Here's how the part is built. I have some questions about the finished solid (model axes, mm). A direction names the side the tool comes from. Coordinates: 2 decimals unless noted, no trailing zeros. Write each loop counter-clockwise with the first axis right and the second up, starting at its lowest first coordinate (ties: lowest second). Pieces come first, ordered by that corner, then holes. Notation, with made-up numbers: (43.25, 26.5) -> (61.25, 26.5) arc R24 cw to (61.25, 43.5) -> close; hole circle Ø4 at (-32.5, 74.25). An arc over 180 degrees is marked (long way). Answer in a Markdown table with one row per item. Add a question column.
from build123d import *

# Parameters (mm, degrees)
BOSS_EXTRUDE1_DEPTH          = 30
EDGE_FLANGE1_STRIP_CUT_DEPTH = 30
EDGE_FLANGE1_DEPTH           = 30
EDGE_FLANGE2_STRIP_CUT_DEPTH = 30
EDGE_FLANGE2_DEPTH           = 30


# Sheet-metal steps are written as plain solids
with BuildPart() as part:
    # Sketch1 → Boss-Extrude1 (new body)
    with BuildSketch(Plane(origin=(0, 0, 0), x_dir=(0, 0, -1), z_dir=(1, 0, 0))):
        Polygon((0.196961551, -0.034729636), (8.879370434, 49.205658015), (8.485447333, 49.275117286), (-0.196961551, 0.034729636), align=None)
    extrude(amount=BOSS_EXTRUDE1_DEPTH)

    # Edge-Flange1 strip (across the edge) → Edge-Flange1 strip cut (cut)
    with BuildSketch(Plane(origin=(30, 49.275117286, -8.485447333), x_dir=(0, 0, 1), z_dir=(-1, 0, 0))):
        Polygon((-0.804601829, 2.259615531), (-0.387846202, -0.103923077), (0.006076899, -0.034463806), (-0.410678728, 2.329074802), align=None)
    extrude(amount=EDGE_FLANGE1_STRIP_CUT_DEPTH, mode=Mode.SUBTRACT)

    # Edge-Flange1 section (across the edge) → Edge-Flange1 (add)
    with BuildSketch(Plane(origin=(30, 49.275117286, -8.485447333), x_dir=(0, 0, 1), z_dir=(-1, 0, 0))):
        with BuildLine():
            Line((-0.4, 0.034995465), (-0.4, 2.965004535))
            Line((-0.4, 2.965004535), (0, 2.965004535))
            Line((0, 2.965004535), (0, 0.034995465))
            ThreePointArc((0, 0.034995465), (0.001522121, 0.000133168), (0.006076899, -0.034463806))
            Line((0.006076899, -0.034463806), (-0.387846202, -0.103923077))
            ThreePointArc((-0.387846202, -0.103923077), (-0.396955758, -0.034729129), (-0.4, 0.034995465))
        make_face()
    extrude(amount=EDGE_FLANGE1_DEPTH)

    # Edge-Flange2 strip (across the edge) → Edge-Flange2 strip cut (cut)
    with BuildSketch(Plane(origin=(30, -0.034729636, -0.196961551), x_dir=(0, 0, -1), z_dir=(-1, 0, 0))):
        Polygon((-0.804601829, 2.259615531), (-0.387846202, -0.103923077), (0.006076899, -0.034463806), (-0.410678728, 2.329074802), align=None)
    extrude(amount=EDGE_FLANGE2_STRIP_CUT_DEPTH, mode=Mode.SUBTRACT)

    # Edge-Flange2 section (across the edge) → Edge-Flange2 (add)
    with BuildSketch(Plane(origin=(30, -0.034729636, -0.196961551), x_dir=(0, 0, -1), z_dir=(-1, 0, 0))):
        with BuildLine():
            Line((-0.4, 0.034995465), (-0.4, 2.965004535))
            Line((-0.4, 2.965004535), (0, 2.965004535))
            Line((0, 2.965004535), (0, 0.034995465))
            ThreePointArc((0, 0.034995465), (0.001522121, 0.000133168), (0.006076899, -0.034463806))
            Line((0.006076899, -0.034463806), (-0.387846202, -0.103923077))
            ThreePointArc((-0.387846202, -0.103923077), (-0.396955758, -0.034729129), (-0.4, 0.034995465))
        make_face()
    extrude(amount=EDGE_FLANGE2_DEPTH)


solid = part.part
Q1. I need wall thicknesses on line 1 (Z direction, x = 2.5, y = 1.5); line 2 (Z direction, x = 18, y = 41). Which ranges of each line are inside material? Lowest first, please. Write a range as [from, to].
Q2. Imagine slicing it at B-B on z = -2.75. Please give me the cut outline in (x, y), plus the area to 3 significant figures.
Q3. Imagine slicing it at C-C on y = 27.5. Please give me the cut outline in (x, z), plus the area to 3 significant figures.
Q4. For faces 1 (the flat face through (15, 51, -8.885)), 2 (the flat face through (15, -2, -0.197)), 3 (the flat face through (15, 51, -8.485)), which set-ups out of +Z, -Z, +X, -X, +Y, -Y let a thin tool reach every point of the face, with its end or its side?
Q5. I'm going to push flat-ended pins straight in: P1, Ø5, axis at x = 4.5, y = 38.5, coming from the -Z side; P2, Ø3, axis at y = 30.5, z = -3, coming from the +X side; P3, Ø0.9, axis at x = 22.5, y = -1, coming from the -Z side; P4, Ø5, axis at x = 18.5, y = 5.5, coming from the +Z side. Where does each tip first touch, or does it pass through?
Q6. Imagine slicing it at A-A on x = 11. Please give me the cut outline in (y, z).
Result sheet:
| question | item | result |
|---|---|---|
| 1 | line 1 | z = [-0.47, -0.06] |
| 1 | line 2 | z = [-7.43, -7.03] |
| 2 | outline | (0, 14.44) -> (30, 14.44) -> (30, 16.75) -> (0, 16.75) -> close |
| 2 | area | 69.1 mm^2 |
| 3 | outline | (0, -5.05) -> (30, -5.05) -> (30, -4.65) -> (0, -4.65) -> close |
| 3 | area | 12.2 mm^2 |
| 4 | face 1 | -Z, +X, -X, +Y, -Y |
| 4 | face 2 | -Z, +X, -X, -Y |
| 4 | face 3 | +Z, +X, -X, +Y |
| 5 | P1 | stops at z = -7.43 |
| 5 | P2 | passes through |
| 5 | P3 | stops at z = -0.2 |
| 5 | P4 | stops at z = -0.33 |
| 6 | outline | (-3, -0.2) -> (-0.07, -0.2) arc R0.4 cw to (0, -0.2) -> (49.17, -8.87) arc R0.8 ccw to (49.31, -8.89) -> (52.24, -8.89) -> (52.24, -8.49) -> (49.31, -8.49) arc R0.4 cw to (49.24, -8.48) -> (0.07, 0.19) arc R0.8 ccw to (-0.07, 0.2) -> (-3, 0.2) -> close |
